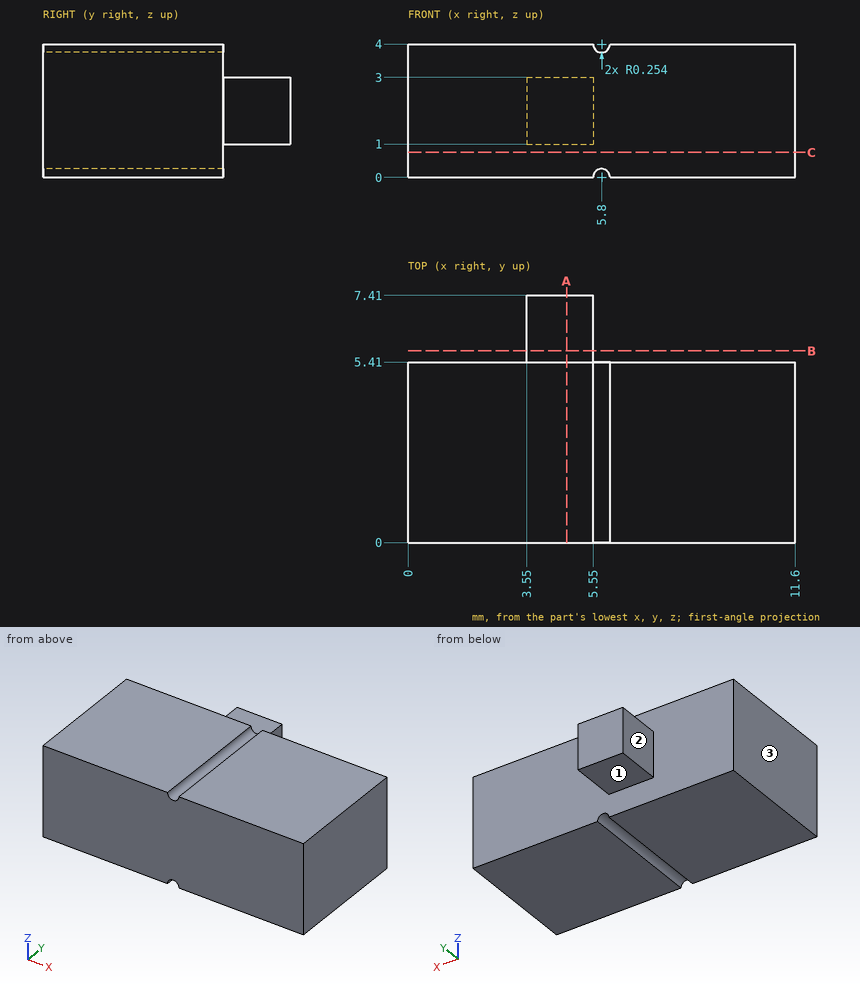
Job drawing, mm, ordinate dimensions from the low corner. One solid piece. A direction names the side the tool comes from. Coordinates: 2 decimals unless noted, no trailing zeros. Loops run counter-clockwise (first coordinate to the right, second up) from the corner with the lowest first, then second, coordinate; pieces in that order, holes last. Notation, with made-up numbers: (-39.5, 11) -> (-23.5, 11) arc R20 cw to (-23.5, 26) -> close; hole circle Ø7 at (3.5, 71.5). An arc over 180 degrees is marked (long way). One line per item, written item: value.
1. Drill centre lines: line 1 (Y direction, x = 1.5, z = 2.1); line 2 (X direction, y = 4, z = 3.85) (1 decimal); line 3 (X direction, y = 5.75, z = 2.45). Where is each one in solid material? Low to high. Write a range as [from, to].
Answers:
line 1: y = [0, 5.41]
line 2: x = [0, 5.6], [6, 11.6]
line 3: x = [3.55, 5.55]
2. Flat gauge pins, fed straight in: P1, Ø1.6, axis at x = 4, y = 7, coming from the -Z side; P2, Ø1, axis at x = 5, y = 6.5, coming from the +Z side; P3, Ø0.6, axis at y = 6.5, z = 1.5, coming from the +X side. Where does each tip first touch, or does it go through?
Answers:
P1: stops at z = 1
P2: stops at z = 3
P3: stops at x = 5.55
3. Slice it at B-B on y = 5.75. Write the cut outline in (x, z).
Answers:
outline: (3.55, 1) -> (5.55, 1) -> (5.55, 3) -> (3.55, 3) -> close
4. Which spindle directions (+Z, -Z, +X, -X, +Y, -Y) get a long thin tool onto all of the face, cutting with end or side? Do the marked faces 1, 2 and 3. Say none if no direction does.
Answers:
face 1: -Z, +X, -X, +Y
face 2: +Z, -Z, -X, +Y
face 3: +Z, -Z, -X, +Y, -Y
5. Slice it at C-C on z = 0.75. Write the cut outline in (x, y).
Answers:
outline: (0, 0) -> (11.6, 0) -> (11.6, 5.41) -> (0, 5.41) -> close
6. Slice it at A-A on x = 4.75. Write the cut outline in (y, z).
Answers:
outline: (0, 0) -> (5.41, 0) -> (5.41, 1) -> (7.41, 1) -> (7.41, 3) -> (5.41, 3) -> (5.41, 4) -> (0, 4) -> close
